Geometry: final body of the model. Coordinates: model frame, mm. A direction names the side the tool comes from. Round coordinates to 2 decimals unless told otherwise and drop trailing zeros. Order: outer loops, then holes, each group sorted by start corner. A loop starts at its lowest first (then second) coordinate and runs counter-clockwise, first axis right, second up. Notation, with made-up numbers: (84.25, -39.75) - (141.25, -39.75) arc R9 ccw to (141.25, -35.75) - close; hole circle Ø6 at (36, -9). An arc over 180 degrees is marked (long way). Put each result on its own line as item: value. Start each with the question number.
(1) Pull-direction query (Y, two-part tool) for faces 1 (the face through (-5.4, 15, 13.9)), 2 (the face through (-4, -8, 10)), 3 (the face through (14, 1, 10)); classes: released by +Y, released by -Y, zero draft, split by the parting line, or undercut.
(2) Section C-C (z = 11.5). Output: boundary loops of the cut face in (x, y).
(3) Section D-D (y = 9). Output: boundary loops of the cut face in (x, z), and give its area (3 significant figures).
(4) Section B-B (x = 3.5). Count the separate pieces of the cut face and the enclosed holes in it, and give its area (3 significant figures).
(5) Access query for faces 4 (the face through (-4, 8, 10)), 5 (the face through (12, 5, 10)), 6 (the face through (17, 5, 10)), 7 (the face through (0.242, 14.485, 2.789)). Directions: +Z, -Z, +X, -X, +Y, -Y. A direction counts if a zero-diameter tool reaches every point of the face in a straight line with its end or side. Return the directions, or none.
(6) Material intervals for L1, parallel to Z at x = 0, y = -13; L2, parallel to Y at x = -3.5, z = 8; L3, parallel to X at y = -12, z = 14, sorted ascending. Write a range as [from, to].
(7) Section A-A (z = 18). Output: boundary loops of the cut face in (x, y).
(8) Pin query (flat end, axial travel): P1, Ø1, axis at y = 10, z = 7, coming from the +X side; P2, Ø2, axis at y = 10, z = 10.5, coming from the -X side; P3, Ø12, axis at x = -8, z = 7.5, coming from the +Y side. Return the tip coordinate at first contact, or that it passes through.
from build123d import *

# Parameters (mm, degrees)
ESBO_O1_W                     = 34.6
ESBO_O1_H                     = 26
RESSALTO_EXTRUS_O1_DEPTH      = 7
ESBO_O10_W                    = 34.6
ESBO_O10_H                    = 2.5
RESSALTO_EXTRUS_O4_DEPTH      = 7
CHANFRO1_SIZE                 = 7
CHANFRO2_SIZE2                = 7
CHANFRO2_SIZE                 = 2.54779164
RESSALTO_EXTRUS_O5_DEPTH      = 15
RESSALTO_EXTRUS_O5_DEPTH_BACK = 15
ESBO_O11_W                    = 16
ESBO_O11_H                    = 14
ESBO_O11_R                    = 5.2
CORTE_EXTRUS_O2_DEPTH         = 1
FILETE1_R                     = 1
RESSALTO_EXTRUS_O6_START      = 12
RESSALTO_EXTRUS_O6_DEPTH      = 5
ESBO_O15_W                    = 19.413269766
ESBO_O15_H                    = 16
CORTE_EXTRUS_O3_DEPTH         = 15


with BuildPart() as part:
    # Esboço1 → Ressalto-extrusão1 (new body)
    with BuildSketch(Plane.XY):
        Rectangle(ESBO_O1_W, ESBO_O1_H)
    extrude(amount=RESSALTO_EXTRUS_O1_DEPTH)

    # Esboço10 → Ressalto-extrusão4 (add)
    with BuildSketch(Plane(origin=(0, 0, 0), x_dir=(-1, 0, 0), z_dir=(0, 0, -1))):
        Polygon((-17.3, -19.5), (0, -26.5), (17.3, -19.5), (17.3, -13), (-17.3, -13), align=None)
        with Locations((0, 14.25)):
            Rectangle(ESBO_O10_W, ESBO_O10_H)
    extrude(amount=-RESSALTO_EXTRUS_O4_DEPTH)

    # Chanfro1
    chanfro1_edges = [part.edges().sort_by_distance(p)[0] for p in [
        (8.65, -23, 7),
        (-8.65, -23, 7),
    ]]
    chamfer(chanfro1_edges, length=CHANFRO1_SIZE - 0.0001)  # a hair under: the kernel refuses the full size

    # Chanfro2
    chanfro2_edges = [part.edges().sort_by_distance(p)[0] for p in [
        (0, 15.5, 7),
    ]]
    chanfro2_side = [part.faces().sort_by_distance(p)[0] for p in [
        (0, 15.449044167, 7),
    ]]
    chamfer(chanfro2_edges, length=CHANFRO2_SIZE - 0.0001, length2=CHANFRO2_SIZE2 - 0.0001, reference=chanfro2_side[0])  # a hair under: the kernel refuses the full size

    # Esboço11 → Ressalto-extrusão5 (add, two sides: drawn at the far end of the back side and taken through both)
    with BuildSketch(Plane(origin=(0, 0, 0), x_dir=(1, 0, 0), z_dir=(0, 1, 0)).offset(-RESSALTO_EXTRUS_O5_DEPTH_BACK)):
        with Locations((0, -14)):
            Rectangle(ESBO_O11_W, ESBO_O11_H)
        with Locations(Location((0, -14, 0), (0, 0, 270))):
            Circle(ESBO_O11_R, mode=Mode.SUBTRACT)
    extrude(amount=RESSALTO_EXTRUS_O5_DEPTH + RESSALTO_EXTRUS_O5_DEPTH_BACK)

    # Esboço13 → Corte-extrusão2 (cut)
    with BuildSketch(Plane.XY.offset(7)):
        Polygon((8, -15), (-8, -15), (-8, 18.845540147), (-17.3, 18.845540147), (-17.3, -24.216996946), (-0.570267535, -24.216996946), (17.3, -21.247378204), (17.3, 18.845540147), (8, 18.845540147), align=None)
    extrude(amount=-CORTE_EXTRUS_O2_DEPTH, mode=Mode.SUBTRACT)

    # Filete1
    filete1_edges = [part.edges().sort_by_distance(p)[0] for p in [
        (0, 12.95230836, 7),
    ]]
    fillet(filete1_edges, radius=FILETE1_R)

    # Esboço14 → Ressalto-extrusão6 (add)
    with BuildSketch(Plane(origin=(0, 0, 0), x_dir=(0, 0, -1), z_dir=(1, 0, 0)).offset(RESSALTO_EXTRUS_O6_START)):
        Polygon((-6, 9.911761874), (-14, 7), (-14, 0), (-13, 0), (-11, 2), (-9, 0), (-6, 0), align=None)
    ressalto_extrus_o6 = extrude(amount=RESSALTO_EXTRUS_O6_DEPTH)

    # Espelhar1: Ressalto-extrusão6 across plane
    add(ressalto_extrus_o6.mirror(Plane(origin=(0, 0, 0), x_dir=(0, 0, 1), z_dir=(1, 0, 0))))

    # Esboço15 → Corte-extrusão3 (cut)
    with BuildSketch(Plane.XY.offset(21)):
        Rectangle(ESBO_O15_W, ESBO_O15_H)
    extrude(amount=-CORTE_EXTRUS_O3_DEPTH, mode=Mode.SUBTRACT)


solid = part.part
Checks:
1. face 1: released by +Y
1. face 2: undercut
1. face 3: released by -Y
2. outline: (-17, 1.5) - (-12, 1.5) - (-12, 7.91) - (-17, 7.91) - close; (-8, -15) - (-4.56, -15) - (-4.56, -8) - (-8, -8) - close; (-8, 8) - (-4.56, 8) - (-4.56, 15) - (-8, 15) - close; (4.56, -15) - (8, -15) - (8, -8) - (4.56, -8) - close; (4.56, 8) - (8, 8) - (8, 15) - (4.56, 15) - close; (12, 1.5) - (17, 1.5) - (17, 7.91) - (12, 7.91) - close
3. outline: (-17.3, 0) - (17.3, 0) - (17.3, 6) - (17, 6) - (17, 8.51) - (12, 8.51) - (12, 6) - (8, 6) - (8, 21) - (-8, 21) - (-8, 6) - (-12, 6) - (-12, 8.51) - (-17, 8.51) - (-17, 6) - (-17.3, 6) - close; hole circle Ø10.4 at (0, 14)
3. area: 388 mm²
4. separate pieces: 3
4. enclosed holes: 0
4. area: 318 mm²
5. face 4: +Z
5. face 5: +Z, +Y, -Y
5. face 6: +Z, +X, +Y, -Y
5. face 7: +X, -X, +Y
6. L1: z = [0, 8.8], [19.2, 21]
6. L2: y = [-15, -8], [8, 15]
6. L3: x = [-8, -5.2], [5.2, 8]
7. outline: (-8, -15) - (-3.32, -15) - (-3.32, -8) - (-8, -8) - close; (-8, 8) - (-3.32, 8) - (-3.32, 15) - (-8, 15) - close; (3.32, -15) - (8, -15) - (8, -8) - (3.32, -8) - close; (3.32, 8) - (8, 8) - (8, 15) - (3.32, 15) - close
8. P1: stops at x = 17
8. P2: stops at x = -8
8. P3: stops at y = 15
